Design review of the part built by this model. Coordinates are the model's own, in mm. Coordinates: 2 decimals unless noted, no trailing zeros. Order: outer loops, then holes, each group sorted by start corner. A loop starts at its lowest first (then second) coordinate and runs counter-clockwise, first axis right, second up. Notation, with made-up numbers: (71.5, 71.5) -> (106.5, 71.5) arc R8 ccw to (106.5, 79.5) -> close; hole circle Ø6 at (70, 60.25). An arc over 180 degrees is marked (long way). Write item = value, one per line.
Autodesk Inventor part; units mm, degrees
ref_plane "YZ Plane" through (0, 0, 0) normal (1, 0, 0) x (0, 1, 0)
ref_plane "XZ Plane" through (0, 0, 0) normal (0, 1, 0) x (-1, 0, 0)
ref_plane "XY Plane" through (0, 0, 0) normal (0, 0, 1) x (1, 0, 0)
sketch "Sketch1" plane through (0, 0, 0) normal (0, 1, 0) x (-1, 0, 0)
  circle A0 centre (0, 0) radius 139.7
  line L0 (-146.05, 146.05) -> (-146.05, -146.05)
  line L1 (-146.05, -146.05) -> (0, -146.05)
  line L2 (-158.75, 158.75) -> (-158.75, -158.75)
  line L3 (-158.75, -158.75) -> (0, -158.75)
  line L4 (0, -158.75) -> (0, -146.05)
  line L5 (-146.05, 146.05) -> (146.05, 146.05)
  line L6 (146.05, 146.05) -> (146.05, 146.05)
  line L7 (146.05, 146.05) -> (158.75, 146.05)
  line L8 (158.75, 146.05) -> (158.75, 158.75)
  line L9 (158.75, 158.75) -> (-158.75, 158.75)
  dimension "d0" = 279.4
  dimension "d2" = 146.05
  dimension "d4" = 146.05
  dimension "d6" = 0
  dimension "d9" = 317.5
  dimension "d30" = 12.7
  dimension "d31" = 292.1
  dimension "d32" = 0
  dimension "d33" = 12.7
  dimension "d34" = 12.7
extrude "Extrusion1" add sketch "Sketch1" along normal blind 6.35 contours L0 L1 L4 L3 L2 L9 L8 L7 L5
sketch "Sketch2" plane through (0, 6.35, 0) normal (0, 1, 0) x (1, 0, 0)
  line L0 (-50.8, -158.75) -> (158.75, -158.75)
  line L1 (158.75, -158.75) -> (158.75, 158.75)
  line L2 (158.75, 158.75) -> (0, 158.75)
  line L3 (146.05, 146.05) -> (146.05, -146.05)
  line L4 (149.225, -149.225) -> (149.225, -155.575)
  line L5 (149.225, -155.575) -> (155.575, -155.575)
  line L6 (155.575, -155.575) -> (155.575, -149.225)
  line L7 (149.225, -149.225) -> (155.575, -149.225)
  line L8 (155.575, 146.05) -> (149.225, 146.05)
  line L9 (149.225, 146.05) -> (149.225, 139.7)
  line L10 (149.225, 139.7) -> (155.575, 139.7)
  line L11 (155.575, 139.7) -> (155.575, 146.05)
  point P0 (0, 0)
  dimension "d12" = 6.35
  dimension "d13" = 6.35
  dimension "d14" = 6.35
  dimension "d15" = 3.175
  dimension "d16" = 3.175
  dimension "d20" = 12.7
  dimension "d22" = 3.175
  dimension "d23" = 6.35
  dimension "d24" = 6.35
extrude "Extrusion2" cut sketch "Sketch2" against normal blind 6.35
sketch "Sketch3" plane through (0, 6.35, 0) normal (0, 1, 0) x (1, 0, 0)
  line L0 (158.75, -158.75) -> (158.75, 158.75)
  line L1 (158.75, 158.75) -> (0, 158.75)
  line L2 (0, 158.75) -> (0, 146.05)
  line L3 (0, 146.05) -> (146.05, 146.05)
  line L4 (146.05, 146.05) -> (146.05, -146.05)
  line L5 (146.05, 146.05) -> (146.05, 149.225)
  line L6 (146.05, 149.225) -> (158.75, 149.225)
  point P0 (0, 0)
  dimension "d27" = 3.175
extrude "Extrusion3" cut sketch "Sketch3" against normal blind 25.4
sketch "Sketch4" plane through (0, 6.35, 0) normal (0, 1, 0) x (1, 0, 0)
  line L0 (-146.05, -146.05) -> (-146.05, 50.8)
  line L1 (146.05, -146.05) -> (-158.75, -146.05)
  line L2 (-158.75, -146.05) -> (-158.75, -158.75)
  line L3 (-158.75, -158.75) -> (158.75, -158.75)
  line L4 (-155.575, -149.225) -> (-149.225, -149.225)
  line L5 (-149.225, -149.225) -> (-149.225, -155.575)
  line L6 (-149.225, -155.575) -> (-155.575, -155.575)
  line L7 (-155.575, -155.575) -> (-155.575, -149.225)
  line L8 (-155.575, -149.225) -> (-149.225, -149.225)
  line L9 (-149.225, -149.225) -> (-149.225, -155.575)
  line L10 (-149.225, -155.575) -> (-155.575, -155.575)
  line L11 (-155.575, -155.575) -> (-155.575, -149.225)
  point P0 (0, 0)
  dimension "d35" = 6.35
  dimension "d36" = 6.35
  dimension "d37" = 3.175
  dimension "d38" = 3.175
  dimension "d39" = 6.35
  dimension "d40" = 6.35
  dimension "d41" = 3.175
  dimension "d42" = 3.175
extrude "Extrusion4" cut sketch "Sketch4" against normal blind 25.4
sketch "Sketch5" plane through (0, 6.35, 0) normal (0, 1, 0) x (1, 0, 0)
  line L0 (146.05, 149.225) -> (146.05, -146.05)
  line L1 (146.05, -146.05) -> (-158.75, -146.05)
  line L2 (15.614, 398.8063) -> (14.3339, 396.1981)
  line L3 (-2.3465, 398.8063) -> (15.614, 398.8063)
  line L4 (-15.5314, 408.5363) -> (-2.3465, 398.8063)
  line L5 (-126.7438, 181.9462) -> (-15.5314, 408.5363)
  line L6 (-126.5217, 145.8051) -> (-126.7438, 181.9462)
  line L7 (-172.6074, 51.9077) -> (-126.5217, 145.8051)
  line L8 (-220.5546, 34.8604) -> (-192.6079, 6.9152)
  line L9 (-192.6079, 6.9152) -> (-161.0476, 38.8664)
  line L10 (-106.2691, 150.4752) -> (-161.0476, 38.8664)
  line L11 (-106.2691, 150.4752) -> (-104.024, 150.4752)
  line L12 (-104.024, 150.4752) -> (-98.9034, 160.9082)
  line L13 (-98.9034, 160.9082) -> (-101.1485, 160.9082)
  line L14 (9.2132, 385.765) -> (-101.1485, 160.9082)
  line L15 (11.4583, 385.765) -> (9.2132, 385.765)
  line L16 (16.5789, 396.1981) -> (11.4583, 385.765)
  line L17 (14.3339, 396.1981) -> (16.5789, 396.1981)
  line L18 (146.05, 23.2231) -> (123.825, -22.0593)
  line L19 (123.825, -22.0593) -> (123.825, -146.05)
  line L20 (-172.6074, 51.9077) -> (-188.2578, 67.5573)
  line L21 (-188.2578, 67.5573) -> (-220.5546, 34.8604)
  point P0 (0, 0)
  dimension "d47" = 22.225
  dimension "d48" = 282.575
extrude "Extrusion5" add sketch "Sketch5" against normal blind 6.35 contours L0 L1 L19 L18
sketch "Sketch6" plane through (0, 6.35, 0) normal (0, 1, 0) x (1, 0, 0)
  line L0 (123.825, -22.0593) -> (123.825, -146.05)
  line L1 (123.825, -146.05) -> (-158.75, -146.05)
  circle A0 centre (136.525, -139.7) radius 3.3782
  circle A1 centre (136.525, -31.75) radius 3.3782
  point P0 (0, 0)
  dimension "d51" = 6.7564
  dimension "d52" = 6.7564
  dimension "d55" = 6.35
  dimension "d56" = 12.7
  dimension "d59" = 12.7
  dimension "d60" = 107.95
extrude "Extrusion6" cut sketch "Sketch6" against normal blind 6.35
properties part number "Bottom Plate" material "Polycarbonate, Clear"
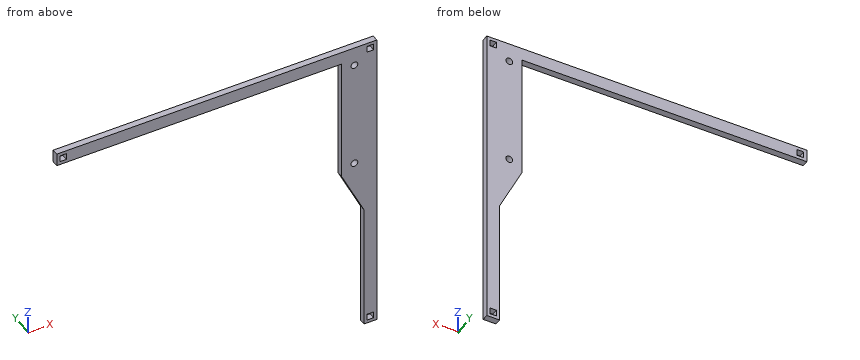
(1) We need section A-A (y = 2.25). Write out the cut boundary in (x, z) (3 decimals), and give its area (3 significant figures).
Report:
outline = (-158.75, 146.05) -> (123.825, 146.05) -> (123.825, 22.059) -> (146.05, -23.223) -> (146.05, -149.225) -> (158.75, -149.225) -> (158.75, 158.75) -> (-158.75, 158.75) -> close; hole (-155.575, 149.225) -> (-149.225, 149.225) -> (-149.225, 155.575) -> (-155.575, 155.575) -> close; hole circle Ø6.756 at (136.525, 31.75); hole circle Ø6.756 at (136.525, 139.7); hole (149.225, -146.05) -> (155.575, -146.05) -> (155.575, -139.7) -> (149.225, -139.7) -> close; hole (149.225, 149.225) -> (155.575, 149.225) -> (155.575, 155.575) -> (149.225, 155.575) -> close
area = 10,800 mm²
(2) For L1, parallel to X at y = 5.5, z = 140 (3 decimals); L2, parallel to X at y = 5, z = 139.7 (3 decimals); L3, parallel to Z at x = -111.5, y = 5.5, list the stretches that pass through material, from the lowest coordinate up.
Report:
L1 = 123.825 to 133.16, 139.89 to 158.75
L2 = 123.825 to 133.147, 139.903 to 158.75
L3 = 146.05 to 158.75
(3) We need section B-B (x = -67). Write out the cut boundary in (y, z), and give its area (3 significant figures).
Report:
outline = (0, 146.05) -> (6.35, 146.05) -> (6.35, 158.75) -> (0, 158.75) -> close
area = 80.6 mm²
(4) Insertion check: pin 1 (1 mm diameter, centred on y = 4.5, z = -86, fed in from -X); pin 2 (1 mm diameter, centred on x = 58.5, y = 5.5, fed in from -Z). Each pin has a flat end and moves straight along its axis. Give the tip position at first contact, or say it passes through.
Report:
pin_1 = 146.05
pin_2 = 146.05
(5) We need section C-C (z = -61). Write out the cut boundary in (x, y).
Report:
outline = (146.05, 0) -> (158.75, 0) -> (158.75, 6.35) -> (146.05, 6.35) -> close
